Solid Edge part; units mm, degrees
sketch "Sketch1" plane through (0, 0, 0) normal (0, -1, 0) x (1, 0, 0)
  circle A0 centre (0, 0) radius 7
  circle A1 centre (0, 0) radius 9
extrude "Protrusion1" add sketch "Sketch1" along normal mid plane 50
sketch "Sketch2" plane through (0, 0, 0) normal (0, 0, 1) x (1, 0, 0)
  circle A0 centre (9.5, 0) radius 1.5
  dimension "D1" = 9.5
revolve "RevolvedCutout1" cut sketch "Sketch2" angle 360 about axis through (0, 54, 0) along (0, -1, 0)
chamfer "Chanfro_2" distance 5 angle 10 2 edges at (-7, -25, 0) (-7, 25, 0) measured on face at (3.8737, -16.1667, 5.8304)
Geometry: final body of the model. Coordinates: model frame, mm. Give positions to 0.01 mm unless a question says otherwise; leave off trailing zeros. Write each loop counter-clockwise with the first axis right and the second up, starting at its lowest first coordinate (ties: lowest second). Pieces come first, ordered by that corner, then holes. Notation, with made-up numbers: (68, -38) - (87, -38) arc R28 ccw to (87, -3) - close; hole circle Ø6 at (85, 19). An arc over 180 degrees is marked (long way). Return JSON: item names as keys, results as strings. Group by question number.
1) Section B-B on x = 0. Return the cut outline in (y, z), plus the area to 3 significant figures.
2) Section C-C on y = -3. Return the cut outline in (x, z).
3) Mould query, pull axis X, two halves, no side actions, for faces 1 (the cylindrical face through (-1.172, -13.042, -8.923)), 2 (the cylindrical face through (6.466, 0.28, 2.681)), 3 (the flat face through (-8, -25, -1)). Classes: released by +X, released by -X, zero draft, split by the parting line, or undercut.
4) Line query: line 1 (Z direction, x = 0, y = -4.5); line 2 (Z direction, x = 1.25, y = 9); line 3 (X direction, y = -2, z = -5.5). Output: solid intervals per line, ascending.
5) First-contact query: P1, Ø1.5, axis at x = -3, y = 16, coming from the +Z side; P2, Ø4, axis at x = -5.5, y = -6, coming from the -Z side; P3, Ø6, axis at x = 4.5, y = -15.5, coming from the +Z side; P4, Ø8, axis at x = -2, z = 0.5, coming from the -Y side. Flat tips, straight axial feed; report the tip coordinate or a pass-through.
6) Section A-A on z = 0. Return the cut outline in (x, y), plus the area to 3 significant figures.
Filled in:
{
 "1": {"outline": "(-25, -9) - (-1.41, -9) arc R1.5 cw to (1.41, -9) - (25, -9) - (25, -7.88) - (20, -7) - (-20, -7) - (-25, -7.88) - close; (-25, 7.88) - (-20, 7) - (20, 7) - (25, 7.88) - (25, 9) - (1.41, 9) arc R1.5 cw to (-1.41, 9) - (-25, 9) - close", "area": "187 mm^2"},
 "2": {"outline": "circle Ø18 at (0, 0); hole circle Ø14 at (0, 0)"},
 "3": {"face 1": "split by the parting line", "face 2": "undercut", "face 3": "zero draft"},
 "4": {"line 1": "z = -9 to -7, 7 to 9", "line 2": "z = -8.91 to -6.89, 6.89 to 8.91", "line 3": "x = -7.12 to -4.33, 4.33 to 7.12"},
 "5": {"P1": "stops at z = 8.71", "P2": "stops at z = -8.29", "P3": "stops at z = 8.87", "P4": "passes through"},
 "6": {"outline": "(-9, -25) - (-7.88, -25) - (-7, -20) - (-7, 20) - (-7.88, 25) - (-9, 25) - (-9, 1.41) arc R1.5 cw to (-9, -1.41) - close; (7, -20) - (7.88, -25) - (9, -25) - (9, -1.41) arc R1.5 cw to (9, 1.41) - (9, 25) - (7.88, 25) - (7, 20) - close", "area": "187 mm^2"}
}
